```python
from build123d import *

# Parameters (mm, degrees)
ESQUISSE1_R        = 2.75
BOSS_EXTRU_1_DEPTH = 3


with BuildPart() as part:
    # Esquisse1 → Boss.-Extru.1 (new body)
    with BuildSketch(Plane.XY):
        Polygon((0, 0), (0, 40), (38, 78), (78, 78), (78, 0), align=None)
        with Locations((9, 29)):
            Circle(ESQUISSE1_R, mode=Mode.SUBTRACT)
        with Locations(Location((9, 9, 0), (0, 0, 180))):
            Circle(ESQUISSE1_R, mode=Mode.SUBTRACT)
        with Locations((29, 9)):
            Circle(ESQUISSE1_R, mode=Mode.SUBTRACT)
        with Locations(Location((29, 29, 0), (0, 0, 180))):
            Circle(ESQUISSE1_R, mode=Mode.SUBTRACT)
        with Locations((49, 29)):
            Circle(ESQUISSE1_R, mode=Mode.SUBTRACT)
        with Locations(Location((49, 9, 0), (0, 0, 180))):
            Circle(ESQUISSE1_R, mode=Mode.SUBTRACT)
        with Locations((69, 9)):
            Circle(ESQUISSE1_R, mode=Mode.SUBTRACT)
        with Locations((69, 29)):
            Circle(ESQUISSE1_R, mode=Mode.SUBTRACT)
        with Locations((49, 49)):
            Circle(ESQUISSE1_R, mode=Mode.SUBTRACT)
        with Locations(Location((69, 49, 0), (0, 0, 180))):
            Circle(ESQUISSE1_R, mode=Mode.SUBTRACT)
        with Locations((69, 69)):
            Circle(ESQUISSE1_R, mode=Mode.SUBTRACT)
        with Locations(Location((49, 69, 0), (0, 0, 180))):
            Circle(ESQUISSE1_R, mode=Mode.SUBTRACT)
    extrude(amount=BOSS_EXTRU_1_DEPTH)


solid = part.part
```
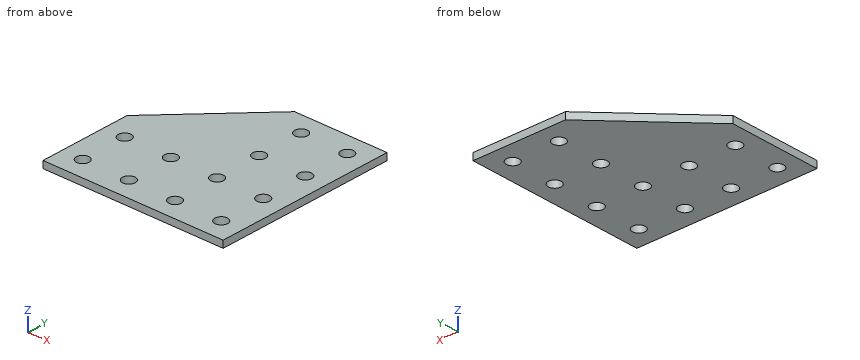
The model under review builds one solid part; all positions refer to its coordinate system, in mm. Give positions to 0.01 mm unless a question says otherwise; leave off trailing zeros. Write each loop counter-clockwise with the first axis right and the second up, starting at its lowest first coordinate (ties: lowest second). Pieces come first, ordered by that corner, then holes. Notation, with made-up numbers: M -28.5,-1.5 L -5.5,-1.5 A28 ccw -5.5,17.5 Z; hole C 23.5,26.25 d9. An arc over 180 degrees is marked long. Write item = value, one per line. Start each with the question number.
Q1. Clearance check with flat-ended pins moving along their axes: pin 1 (5 mm diameter, centred on x = 9, y = 29, fed in from -Z); pin 2 (1 mm diameter, centred on y = 64.5, z = 1.5, fed in from -X). State where each tip first meets the part, or that it passes through.
Q2. We need section B-B (y = 9). State the section outline as (x, z) points.
Q3. We need section D-D (y = 49). State the section outline as (x, z) points.
Q4. For line 1 (Y direction, x = 69, z = 1.9); line 2 (Y direction, x = 26.5, z = 1.95); line 3 (Y direction, x = 6.5, z = 2.65), list the stretches that pass through material, from the lowest coordinate up.
Q5. We need section A-A (x = 29). State the section outline as (y, z) points, plus the area to 3 significant figures.
Result set:
q1.pin_1 = through
q1.pin_2 = 24
q2.outline = M 0,0 L 6.25,0 L 6.25,3 L 0,3 Z; M 11.75,0 L 26.25,0 L 26.25,3 L 11.75,3 Z; M 31.75,0 L 46.25,0 L 46.25,3 L 31.75,3 Z; M 51.75,0 L 66.25,0 L 66.25,3 L 51.75,3 Z; M 71.75,0 L 78,0 L 78,3 L 71.75,3 Z
q3.outline = M 9,0 L 46.25,0 L 46.25,3 L 9,3 Z; M 51.75,0 L 66.25,0 L 66.25,3 L 51.75,3 Z; M 71.75,0 L 78,0 L 78,3 L 71.75,3 Z
q4.line_1 = 0 to 6.25, 11.75 to 26.25, 31.75 to 46.25, 51.75 to 66.25, 71.75 to 78
q4.line_2 = 0 to 7.85, 10.15 to 27.85, 30.15 to 66.5
q4.line_3 = 0 to 7.85, 10.15 to 27.85, 30.15 to 46.5
q5.outline = M 0,0 L 6.25,0 L 6.25,3 L 0,3 Z; M 11.75,0 L 26.25,0 L 26.25,3 L 11.75,3 Z; M 31.75,0 L 69,0 L 69,3 L 31.75,3 Z
q5.area = 174 mm2
